Source: CAD feature listing. Evaluate the final solid. Frame: model axes, mm. Face numbers are marked on the shaded views. A direction names the side the tool comes from. Give positions to 0.01 mm unless a question says otherwise; leave off trailing zeros. Write each loop counter-clockwise with the first axis right and the second up, starting at its lowest first coordinate (ties: lowest second). Pieces come first, ordered by that corner, then holes. Notation, with made-up numbers: M -13.5,74.25 L 16.5,74.25 A15 ccw 16.5,79.25 Z; hole C -5.5,77 d3. An arc over 180 degrees is marked long. Return JSON: item names as keys, results as strings.
```python
from build123d import *

# Parameters (mm, degrees)
SKETCH1_W       = 40.6
SKETCH1_H       = 33.6
EXTRUDE6_DEPTH  = 20
SKETCH7_R       = 1.93
EXTRUDE12_DEPTH = 46.510692117
SKETCH12_R      = 2
SKETCH12_R_2    = 1.5
EXTRUDE13_DEPTH = 15
SKETCH13_R      = 3
EXTRUDE14_DEPTH = 14.2


with BuildPart() as part:
    # Sketch1 → Extrude6 (new body)
    with BuildSketch(Plane(origin=(0, 0, 0), x_dir=(1, 0, 0), z_dir=(0, 1, 0))):
        with Locations((13.300799804, -6.485389185)):
            Rectangle(SKETCH1_W, SKETCH1_H)
    extrude(amount=EXTRUDE6_DEPTH)

    # Sketch7 → Extrude12 (cut, through all)
    with BuildSketch(Plane(origin=(0, 20, 0), x_dir=(-1, 0, 0), z_dir=(0, 1, 0))):
        with Locations(Location((-1.385799804, -6.619610815, 0), (0, 0, 90))):
            Circle(SKETCH7_R)
        with Locations(Location((-25.215799804, -6.619610815, 0), (0, 0, 90))):
            Circle(SKETCH7_R)
        with Locations(Location((-1.385799804, 19.590389185, 0), (0, 0, 90))):
            Circle(SKETCH7_R)
        with Locations(Location((-25.215799804, 19.590389185, 0), (0, 0, 90))):
            Circle(SKETCH7_R)
    extrude(amount=-EXTRUDE12_DEPTH, mode=Mode.SUBTRACT)

    # Sketch12 → Extrude13 (cut)
    with BuildSketch(Plane(origin=(0, 20, 0), x_dir=(1, 0, 0), z_dir=(0, 1, 0))):
        with Locations(Location((7.200799804, -6.485389185, 0), (0, 0, 270))):
            Circle(SKETCH12_R)
        with Locations(Location((13.300799804, -0.385389185, 0), (0, 0, 270))):
            Circle(SKETCH12_R_2)
        with Locations(Location((19.400799804, -6.485389185, 0), (0, 0, 270))):
            Circle(SKETCH12_R)
        with Locations(Location((13.300799804, -12.585389185, 0), (0, 0, 270))):
            Circle(SKETCH12_R_2)
    extrude(amount=-EXTRUDE13_DEPTH, mode=Mode.SUBTRACT)

    # Sketch13 → Extrude14 (cut)
    with BuildSketch(Plane(origin=(33.600799804, 0, 0), x_dir=(0, 0, -1), z_dir=(1, 0, 0))):
        with Locations((-6.485389185, 10)):
            Circle(SKETCH13_R)
    extrude(amount=-EXTRUDE14_DEPTH, mode=Mode.SUBTRACT)


solid = part.part
```
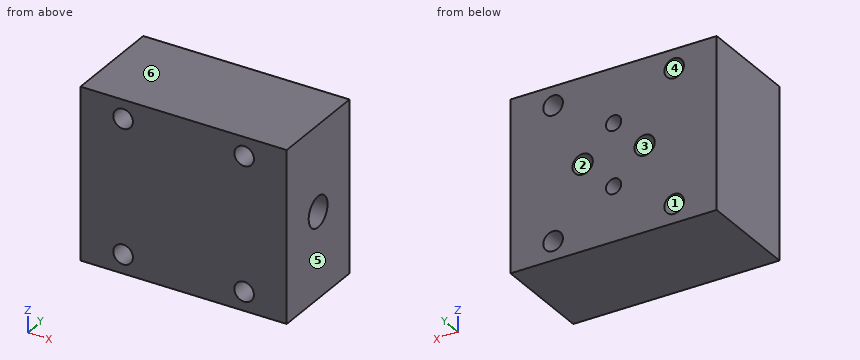
1) Draft query along X for the marked faces 3, 4, 5 and 6. Return one class per face: released by +X, released by -X, zero draft, split by the parting line, or undercut.
Numbers:
{"face 3": "undercut", "face 4": "undercut", "face 5": "released by +X", "face 6": "zero draft"}
2) Contact query for flat-ended pins moving along their axis: pin 1 Ø3.5 at (x, z) = (13.3, 12.59) entering from +Y; pin 2 Ø0.9 at (x, z) = (14, 12.5) entering from +Y. Output: stop coordinate, or through.
Numbers:
{"pin 1": "stops at y = 20", "pin 2": "stops at y = 5"}
3) Cut plane C-C, the plane x = 12.5. Return the cut outline in (y, z), then the cut area to 3 significant figures.
Numbers:
{"outline": "M 0,-10.31 L 20,-10.31 L 20,-0.88 L 5,-0.88 L 5,1.65 L 20,1.65 L 20,11.32 L 5,11.32 L 5,13.85 L 20,13.85 L 20,23.29 L 0,23.29 Z", "area": "596 mm²"}
4) Set-up query: the marked faces 1 and 2. Return all of +Z, -Z, +X, -X, +Y, -Y with unobstructed straight access to the full face (end or side cutting, diameter ignored); none if empty.
Numbers:
{"face 1": "+Y, -Y", "face 2": "+Y"}
5) Line query: line 1 (Z direction, x = 28.75, y = 10); line 2 (X direction, y = 14, z = 18.5); line 3 (Z direction, x = 26, y = 5.75). Output: solid intervals per line, ascending. Write a range as [from, to].
Numbers:
{"line 1": "z = [-10.31, 3.49], [9.49, 23.29]", "line 2": "x = [-7, -0.21], [2.98, 23.62], [26.81, 33.6]", "line 3": "z = [-10.31, -8.38], [-4.86, 17.83], [21.35, 23.29]"}
6) Cut plane B-B, the plane y = 10. Return the cut outline in (x, z).
Numbers:
{"outline": "M -7,-10.31 L 33.6,-10.31 L 33.6,3.49 L 19.4,3.49 L 19.4,4.49 A2 cw 19.4,8.49 L 19.4,9.49 L 33.6,9.49 L 33.6,23.29 L -7,23.29 Z; hole C 1.39,-6.62 d3.86; hole C 1.39,19.59 d3.86; hole C 7.2,6.49 d4; hole C 13.3,0.39 d3; hole C 13.3,12.59 d3; hole C 25.22,-6.62 d3.86; hole C 25.22,19.59 d3.86"}
7) Cut plane A-A, the plane z = -5.5. Return the cut outline in (x, y), then the cut area to 3 significant figures.
Numbers:
{"outline": "M -7,0 L -0.19,0 L -0.19,20 L -7,20 Z; M 2.96,0 L 23.64,0 L 23.64,20 L 2.96,20 Z; M 26.79,0 L 33.6,0 L 33.6,20 L 26.79,20 Z", "area": "686 mm²"}
